from build123d import *

# Parameters (mm, degrees)
SKETCH_1_W          = 10
SKETCH_1_H          = 10
EXTRUDE_1_DEPTH     = 6
SKETCH_2_R          = 1.5
CUT_EXTRUDE_1_DEPTH = 16.362291496
SKETCH_3_R          = 1.5
CUT_EXTRUDE_2_DEPTH = 16.362291496
SKETCH_4_R          = 1.5
CUT_EXTRUDE_3_DEPTH = 16.362291496


with BuildPart() as part:
    # 草图1 → 凸台-拉伸1 (new body)
    with BuildSketch(Plane.XY):
        with Locations((5, 5)):
            Rectangle(SKETCH_1_W, SKETCH_1_H)
    extrude(amount=EXTRUDE_1_DEPTH)

    # 草图2 → 切除-拉伸1 (cut, through all)
    with BuildSketch(Plane(origin=(0, 0, 0), x_dir=(-1, 0, 0), z_dir=(0, 0, -1))):
        with Locations((-5, 5)):
            Circle(SKETCH_2_R)
    extrude(amount=-CUT_EXTRUDE_1_DEPTH, mode=Mode.SUBTRACT)

    # 草图3 → 切除-拉伸2 (cut, through all)
    with BuildSketch(Plane(origin=(0, 10, 0), x_dir=(1, 0, 0), z_dir=(0, 1, 0))):
        with Locations(Location((5, -3, 0), (0, 0, 180))):
            Circle(SKETCH_3_R)
    extrude(amount=-CUT_EXTRUDE_2_DEPTH, mode=Mode.SUBTRACT)

    # 草图4 → 切除-拉伸3 (cut, through all)
    with BuildSketch(Plane.ZY):
        with Locations((3, 5)):
            Circle(SKETCH_4_R)
    extrude(amount=-CUT_EXTRUDE_3_DEPTH, mode=Mode.SUBTRACT)


solid = part.part
Read the model definition and answer for the solid it produces. Units are mm, in the model's axes. Give positions to 0.01 mm unless a question says otherwise; leave off trailing zeros. Write each loop counter-clockwise with the first axis right and the second up, starting at its lowest first coordinate (ties: lowest second). Pieces come first, ordered by that corner, then holes. Notation, with made-up numbers: (39.25, 14) -> (72.25, 14) arc R7 cw to (72.25, 24) -> close; hole circle Ø11 at (14, -18). An arc over 180 degrees is marked (long way). Answer as a JSON object with one key per item and string values. Group by question number.
1) Find section C-C (y = 2.5). Write down the section's boundary in (x, z), and give its area (3 significant figures).
2) Find section D-D (z = 0.55). Write down the section's boundary in (x, y).
3) Consider L1, parallel to X at y = 5, z = 5; L2, parallel to Z at x = 8.3, y = 5. Determine where each line is inside the solid, lowest interval first. Write a range as from..to.
4) The mould has two halves that part along X. Classify faces 1 (the flat face through (0, 6, 1.6)), 2 (the flat face through (10, 6, 1.6)), 3 (the cylindrical face through (6.11, 6.01, 0.74)), 4 (the cylindrical face through (1.94, 6.01, 1.89)): +X half, -X half, draft (parallel to the pull), parting line (faces both ways), or undercut.
5) Find section B-B (z = 3). Write down the section's boundary in (x, y), and give its area (3 significant figures).
6) Find section A-A (x = 5). Write down the section's boundary in (y, z), and give its area (3 significant figures).
Values follow:
{
 "1": {"outline": "(0, 0) -> (10, 0) -> (10, 6) -> (0, 6) -> close; hole circle Ø3 at (5, 3)", "area": "52.9 mm2"},
 "2": {"outline": "(0, 0) -> (10, 0) -> (10, 10) -> (0, 10) -> close; hole circle Ø3 at (5, 5)"},
 "3": {"L1": "x = 0..3.5, 6.5..10", "L2": "z = 0..1.5, 4.5..6"},
 "4": {"face 1": "-X half", "face 2": "+X half", "face 3": "undercut", "face 4": "draft"},
 "5": {"outline": "(0, 0) -> (3.5, 0) -> (3.5, 3.5) -> (0, 3.5) -> close; (0, 6.5) -> (3.5, 6.5) -> (3.5, 10) -> (0, 10) -> close; (6.5, 0) -> (10, 0) -> (10, 3.5) -> (6.5, 3.5) -> close; (6.5, 6.5) -> (10, 6.5) -> (10, 10) -> (6.5, 10) -> close", "area": "49.0 mm2"},
 "6": {"outline": "(0, 0) -> (3.5, 0) -> (3.5, 1.5) -> (0, 1.5) -> close; (0, 4.5) -> (3.5, 4.5) -> (3.5, 6) -> (0, 6) -> close; (6.5, 0) -> (10, 0) -> (10, 1.5) -> (6.5, 1.5) -> close; (6.5, 4.5) -> (10, 4.5) -> (10, 6) -> (6.5, 6) -> close", "area": "21.0 mm2"}
}
